Geometry check sheet. Reference: the model listing, model coordinates, mm. A direction names the side the tool comes from. Give positions to 0.01 mm unless a question says otherwise; leave off trailing zeros. Order: outer loops, then holes, each group sorted by start corner. A loop starts at its lowest first (then second) coordinate and runs counter-clockwise, first axis right, second up.
from build123d import *

# Parameters (mm, degrees)
SKETCH1_W           = 25.4
SKETCH1_H           = 25.4
SKETCH1_W_2         = 19.05
SKETCH1_H_2         = 19.05
EXTRUDE_THIN1_DEPTH = 25.4
SKETCH2_R           = 2.413
CUT_EXTRUDE1_DEPTH  = 26.4


with BuildPart() as part:
    # Sketch1 → Extrude-Thin1 (new body)
    with BuildSketch(Plane(origin=(0, 0, 0), x_dir=(0, 0, -1), z_dir=(1, 0, 0))):
        with Locations((12.7, 12.7)):
            Rectangle(SKETCH1_W, SKETCH1_H)
        with Locations((12.7, 12.7)):
            Rectangle(SKETCH1_W_2, SKETCH1_H_2, mode=Mode.SUBTRACT)
    extrude(amount=EXTRUDE_THIN1_DEPTH)

    # Sketch2 → Cut-Extrude1 (cut, through all)
    with BuildSketch(Plane.XY):
        with Locations((12.7, 12.7)):
            Circle(SKETCH2_R)
    extrude(amount=-CUT_EXTRUDE1_DEPTH, mode=Mode.SUBTRACT)


solid = part.part
Item 1: Sectioned sample at C-C (y = 12.7). Enter the section's corners in (x, z) (3 decimals).
Reported:
outline: (0, -25.4) - (10.287, -25.4) - (10.287, -22.225) - (0, -22.225) - close; (0, -3.175) - (10.287, -3.175) - (10.287, 0) - (0, 0) - close; (15.113, -25.4) - (25.4, -25.4) - (25.4, -22.225) - (15.113, -22.225) - close; (15.113, -3.175) - (25.4, -3.175) - (25.4, 0) - (15.113, 0) - close
Item 2: Sectioned sample at B-B (z = -19.75). Enter the section's corners in (x, y) (3 decimals), and give its area (3 significant figures).
Reported:
outline: (0, 0) - (25.4, 0) - (25.4, 3.175) - (0, 3.175) - close; (0, 22.225) - (25.4, 22.225) - (25.4, 25.4) - (0, 25.4) - close
area: 161 mm2
Item 3: Sectioned sample at D-D (x = 11.5). Enter the section's corners in (y, z) (3 decimals).
Reported:
outline: (0, -25.4) - (10.607, -25.4) - (10.607, -22.225) - (3.175, -22.225) - (3.175, -3.175) - (10.607, -3.175) - (10.607, 0) - (0, 0) - close; (14.793, -25.4) - (25.4, -25.4) - (25.4, 0) - (14.793, 0) - (14.793, -3.175) - (22.225, -3.175) - (22.225, -22.225) - (14.793, -22.225) - close
Item 4: Draft check along Z on faces 3 (the flat face through (25.4, 13, -24)), 4 (the flat face through (12.5, 15.3, 0)), 5 (the flat face through (13, 22.225, -13)). Enter one of: released by +Z, released by -Z, zero draft, split by the parting line, or undercut.
Reported:
face 3: zero draft
face 4: released by +Z
face 5: undercut
Item 5: Set-up check for faces 1 (the flat face through (12.5, 15.3, -25.4)), 2 (the flat face through (13, 3.175, -13)): record each of +Z, -Z, +X, -X, +Y, -Y from which the full face is reachable in a straight line by a thin tool's end or side.
Reported:
face 1: -Z, +X, -X, +Y, -Y
face 2: +X, -X
Item 6: Sectioned sample at A-A (y = 19). Enter the section's corners in (x, z) (3 decimals).
Reported:
outline: (0, -25.4) - (25.4, -25.4) - (25.4, -22.225) - (0, -22.225) - close; (0, -3.175) - (25.4, -3.175) - (25.4, 0) - (0, 0) - close
Item 7: Scan lines: L1, parallel to Z at x = 16, y = 21.5 (3 decimals); L2, parallel to Y at x = 21, z = -16 (3 decimals); L3, parallel to Y at x = 12.7, z = -24.15. Record each from-to range of solid material in increasing order.
Reported:
L1: z = -25.4 to -22.225, -3.175 to 0
L2: y = 0 to 3.175, 22.225 to 25.4
L3: y = 0 to 10.29, 15.11 to 25.4
